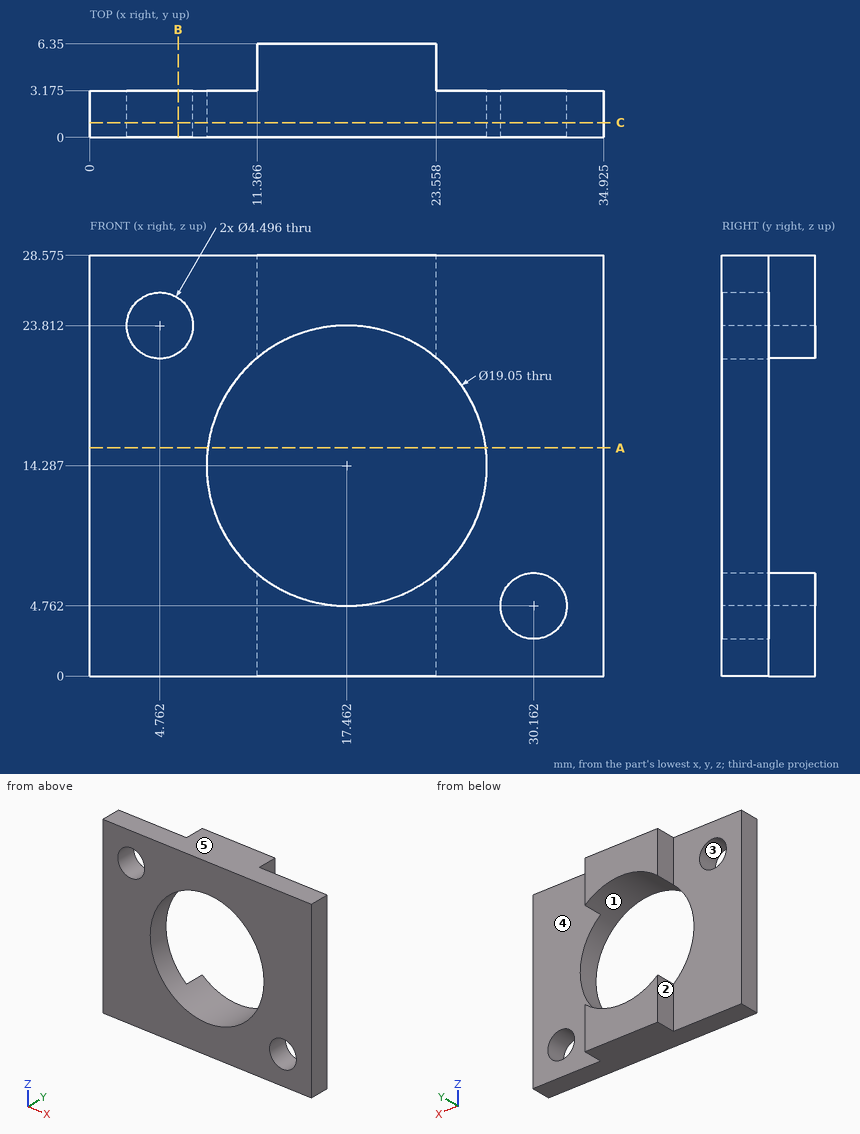
Source: three-view drawing plus pictorial views. Frame: mm from the lowest corner of the part. A direction names the side the tool comes from. Round coordinates to 2 decimals unless told otherwise and drop trailing zeros. Order: outer loops, then holes, each group sorted by start corner. A loop starts at its lowest first (then second) coordinate and runs counter-clockwise, first axis right, second up. Notation, with made-up numbers: (-1, 6.5) - (43, 6.5) arc R37 cw to (43, 42.5) - close; hole circle Ø4 at (4.25, 82.5). An arc over 180 degrees is marked (long way). Use a Markdown table: item, result.
1. Material intervals for probe 1 along X at (y, z) = (1.5, 7.5) (1 decimal); probe 2 along Z at (x, y) = (29, 1) (1 decimal); probe 3 along Y at (x, z) = (29.5, 17.5) (1 decimal), sorted ascending.
Evaluation:
| item | result |
|---|---|
| probe 1 | 0 to 10.8, 24.1 to 34.9 |
| probe 2 | 0 to 2.8, 6.7 to 28.6 |
| probe 3 | 0 to 3.2 |
2. Mould query, pull axis Z, two halves, no side actions, for the marked faces 3, 4 and 5. Classes: +Z half, -Z half, draft (parallel to the pull), parting line (faces both ways), or undercut.
Evaluation:
| item | result |
|---|---|
| face 3 | undercut |
| face 4 | draft |
| face 5 | +Z half |
3. First-contact query: pin 1 (1 mm diameter, centred on y = 4, z = 4, fed in from +X); pin 2 (6 mm diameter, centred on x = 4.76, z = 23.81, fed in from +Y) (1 decimal); pin 3 (3.5 mm diameter, centred on y = 5, z = 3.5, fed in from -X). Flat tips, straight axial feed; report the tip coordinate or a pass-through.
Evaluation:
| item | result |
|---|---|
| pin 1 | x = 23.56 |
| pin 2 | y = 3.2 |
| pin 3 | x = 11.37 |
4. Section C-C on y = 1. State how many separate pieces and enclosed holes the cut face has, then the cut area to 3 significant figures.
Evaluation:
| item | result |
|---|---|
| separate pieces | 1 |
| enclosed holes | 3 |
| area | 681 mm^2 |
5. Section B-B on x = 6. Return the cut outline in (y, z) (1 decimal).
Evaluation:
| item | result |
|---|---|
| outline | (0, 0) - (3.2, 0) - (3.2, 21.9) - (0, 21.9) - close; (0, 25.7) - (3.2, 25.7) - (3.2, 28.6) - (0, 28.6) - close |
6. Section A-A on z = 15.5. Return the cut outline in (x, y) (1 decimal), then the cut area to 3 significant figures.
Evaluation:
| item | result |
|---|---|
| outline | (0, 0) - (8, 0) - (8, 3.2) - (0, 3.2) - close; (26.9, 0) - (34.9, 0) - (34.9, 3.2) - (26.9, 3.2) - close |
| area | 50.9 mm^2 |
7. Access query for the marked faces 1 and 2. Directions: +Z, -Z, +X, -X, +Y, -Y. A direction counts if a zero-diameter tool reaches every point of the face in a straight line with its end or side. Return the directions, or none.
Evaluation:
| item | result |
|---|---|
| face 1 | +Y, -Y |
| face 2 | +Z, -Z, -X, +Y |
